Verification items for this drawing (mm, ordinates from the low corner). A direction names the side the tool comes from. Give positions to 0.01 mm unless a question says otherwise; leave off trailing zeros. Write each loop counter-clockwise with the first axis right and the second up, starting at its lowest first coordinate (ties: lowest second). Pieces come first, ordered by that corner, then holes. Notation, with made-up numbers: (-28, 85.25) -> (10, 85.25) arc R26 cw to (10, 120.25) -> close; hole circle Ø4 at (69.25, 3). An arc over 180 degrees is marked (long way). Use one line per item in the form item = value. Start each with the question number.
(1) Section check B-B, the plane z = 8.25. Record the cut outline in (x, y), plus the area to 3 significant figures.
(2) Section check A-A, the plane x = 15. Record the cut outline in (y, z).
(3) Section check D-D, the plane z = 5. Record the cut outline in (x, y).
(4) Release check for a two-part mould opening along X. For the marked faces 1, 2 and 3 record: pulls with the +X half, pulls with the -X half, needs draft (parallel to the pull), parting line crosses it, or undercut.
(5) Section check C-C, the plane y = 2. Record the cut outline in (x, z).
(6) Depth check by flat-ended pin: pin 1 Ø2 at (y, z) = (22, 6.5) entering from +X; pin 2 Ø2 at (x, y) = (6, 14) entering from -Z; pin 3 Ø3 at (y, z) = (15, 2) entering from +X. Enter the tip coordinate at first touch or a pass-through.
(7) Scan lines: L1, parallel to Y at x = 15, z = 9.7; L2, parallel to X at y = 15, z = 1.95; L3, parallel to Z at x = 10.75, y = 15. Record each from-to range of solid material in increasing order.
(8) Set-up check for the marked faces 4, 5 and 6: record each of +Z, -Z, +X, -X, +Y, -Y from which the full face is reachable in a straight line by a thin tool's end or side.
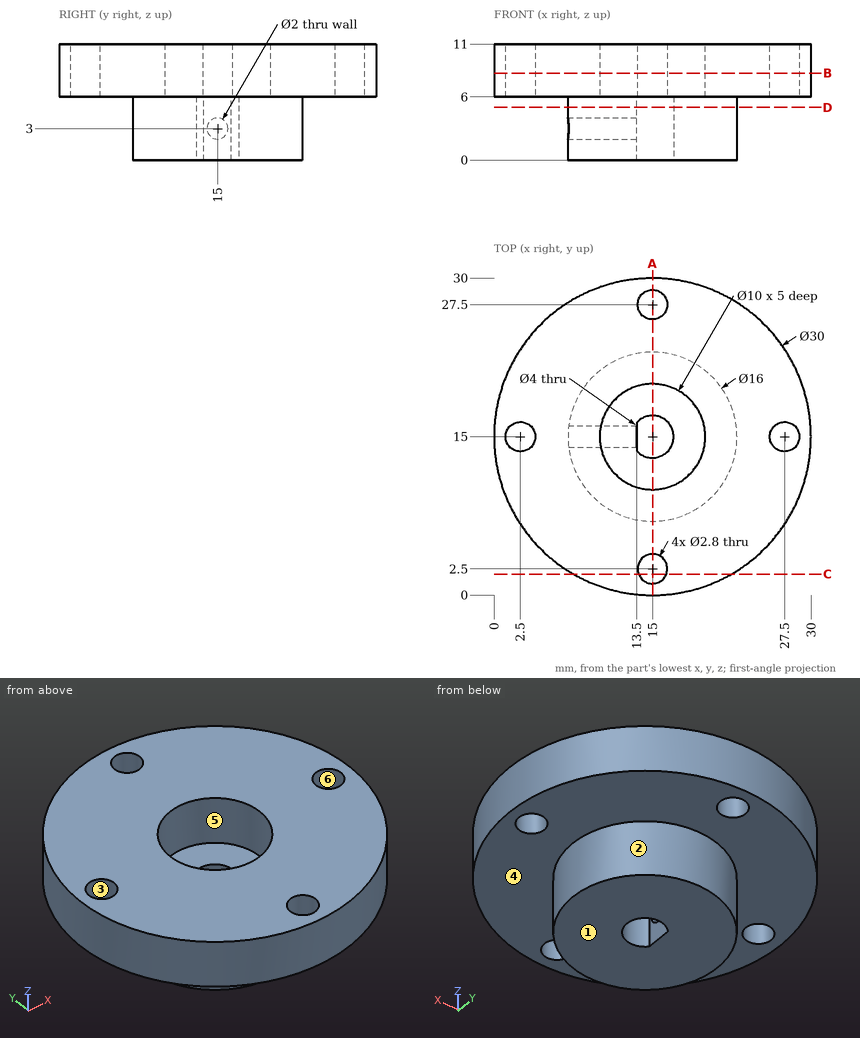
Completed:
q1.outline = circle Ø30 at (15, 15); hole circle Ø2.8 at (2.5, 15); hole circle Ø10 at (15, 15); hole circle Ø2.8 at (15, 2.5); hole circle Ø2.8 at (15, 27.5); hole circle Ø2.8 at (27.5, 15)
q1.area = 604 mm²
q2.outline = (0, 6) -> (1.1, 6) -> (1.1, 11) -> (0, 11) -> close; (3.9, 6) -> (7, 6) -> (7, 0) -> (13, 0) -> (13, 6) -> (10, 6) -> (10, 11) -> (3.9, 11) -> close; (17, 0) -> (23, 0) -> (23, 6) -> (26.1, 6) -> (26.1, 11) -> (20, 11) -> (20, 6) -> (17, 6) -> close; (28.9, 6) -> (30, 6) -> (30, 11) -> (28.9, 11) -> close
q3.outline = circle Ø16 at (15, 15); hole (13.5, 13.68) arc R2 ccw (long way) to (13.5, 16.32) -> close
q4.face_1 = needs draft
q4.face_2 = parting line crosses it
q4.face_3 = undercut
q5.outline = (7.52, 6) -> (13.69, 6) -> (13.69, 11) -> (7.52, 11) -> close; (16.31, 6) -> (22.48, 6) -> (22.48, 11) -> (16.31, 11) -> close
q6.pin_1 = 28.75
q6.pin_2 = 6
q6.pin_3 = 23
q7.L1 = 0 to 1.1, 3.9 to 10, 20 to 26.1, 28.9 to 30
q7.L2 = 7 to 13.5, 17 to 23
q7.L3 = 0 to 2, 4 to 6
q8.face_4 = -Z
q8.face_5 = +Z
q8.face_6 = +Z, -Z
